The listing builds one solid part. Answer for the finished solid, in the listing's coordinates (mm). Coordinates: 2 decimals unless noted, no trailing zeros. Order: outer loops, then holes, each group sorted by start corner. A loop starts at its lowest first (then second) coordinate and runs counter-clockwise, first axis right, second up. Notation, with made-up numbers: (5.5, 81.25) -> (15.5, 81.25) arc R9 ccw to (15.5, 95.25) -> close; hole circle Ø3 at (61, 82.25). An arc over 180 degrees is marked (long way). Answer in a Markdown table with one row per item.
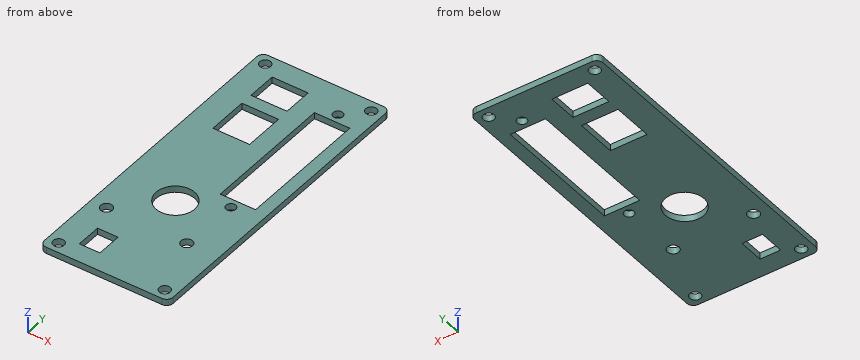
```python
from build123d import *

# Parameters (mm, degrees)
SKETCH_W      = 40
SKETCH_H      = 96.5
PAD_DEPTH     = 2
SKETCH001_R   = 1.7
SKETCH001_R_2 = 1.5
SKETCH001_R_3 = 6
SKETCH001_R_4 = 1.8
SKETCH001_W   = 11
SKETCH001_H   = 41
SKETCH001_W_2 = 11.2
SKETCH001_H_2 = 9.2
SKETCH001_W_3 = 11.4
SKETCH001_H_3 = 12.6
SKETCH001_W_4 = 6.4
SKETCH001_H_4 = 7.9
POCKET_DEPTH  = 5
FILLET_R      = 2
FILLET001_R   = 2
FILLET002_R   = 2
FILLET003_R   = 2


with BuildPart() as part:
    # Sketch → Pad (new body)
    with BuildSketch(Plane.XY):
        Rectangle(SKETCH_W, SKETCH_H)
    extrude(amount=PAD_DEPTH)

    # Sketch001 (on Face6 of Pad) → Pocket (cut)
    with BuildSketch(Plane.XY.offset(2)):
        with Locations((-16.5, 44.95)):
            Circle(SKETCH001_R)
        with Locations((16.5, 44.95)):
            Circle(SKETCH001_R)
        with Locations((-16.5, -44.95)):
            Circle(SKETCH001_R)
        with Locations((16.5, -44.95)):
            Circle(SKETCH001_R)
        with Locations((10.5, 38.85)):
            Circle(SKETCH001_R_2)
        with Locations((10.5, -7.75)):
            Circle(SKETCH001_R_2)
        with Locations((-2.5, -13.75)):
            Circle(SKETCH001_R_3)
        with Locations((-15, -26.25)):
            Circle(SKETCH001_R_4)
        with Locations((10, -26.25)):
            Circle(SKETCH001_R_4)
        with Locations((10.68, 15.55)):
            Rectangle(SKETCH001_W, SKETCH001_H)
        with Locations((-6.4, 37.05754)):
            Rectangle(SKETCH001_W_2, SKETCH001_H_2)
        with Locations((-6.3, 22.205288)):
            Rectangle(SKETCH001_W_3, SKETCH001_H_3)
        with Locations((-8.8, -38.3)):
            Rectangle(SKETCH001_W_4, SKETCH001_H_4)
    extrude(amount=-POCKET_DEPTH, mode=Mode.SUBTRACT)

    # Fillet
    fillet_edges = [part.edges().sort_by_distance(p)[0] for p in [
        (-20, 48.25, 1),
    ]]
    fillet(fillet_edges, radius=FILLET_R)

    # Fillet001
    fillet001_edges = [part.edges().sort_by_distance(p)[0] for p in [
        (20, 48.25, 1),
    ]]
    fillet(fillet001_edges, radius=FILLET001_R)

    # Fillet002
    fillet002_edges = [part.edges().sort_by_distance(p)[0] for p in [
        (-20, -48.25, 1),
    ]]
    fillet(fillet002_edges, radius=FILLET002_R)

    # Fillet003
    fillet003_edges = [part.edges().sort_by_distance(p)[0] for p in [
        (20, -48.25, 1),
    ]]
    fillet(fillet003_edges, radius=FILLET003_R)


solid = part.part
```
(1) A cutting plane is placed at C-C, the plane x = 2. Determine the outline of the cut face in (y, z), then the cut area to 3 significant figures.
Check values:
| item | result |
|---|---|
| outline | (-48.25, 0) -> (-17.72, 0) -> (-17.72, 2) -> (-48.25, 2) -> close; (-9.78, 0) -> (48.25, 0) -> (48.25, 2) -> (-9.78, 2) -> close |
| area | 177 mm² |
(2) A cutting plane is placed at A-A, the plane y = 44.95. Determine the outline of the cut face in (x, z).
Check values:
| item | result |
|---|---|
| outline | (-20, 0) -> (-18.2, 0) -> (-18.2, 2) -> (-20, 2) -> close; (-14.8, 0) -> (14.8, 0) -> (14.8, 2) -> (-14.8, 2) -> close; (18.2, 0) -> (20, 0) -> (20, 2) -> (18.2, 2) -> close |
(3) A cutting plane is placed at D-D, the plane z = 1.1. Count the separate pieces of the cut face and the enclosed holes in it, then the cut area to 3 significant figures.
Check values:
| item | result |
|---|---|
| separate pieces | 1 |
| enclosed holes | 13 |
| area | 2,920 mm² |
(4) Find the intervals of material crossed by line 1 along X through (y, z) = (22, 1.7); line 2 along Y through (x, z) = (-2.5, 0.7); line 3 along Y through (x, z) = (-9.5, 1.95), in increasing order. Write a range as from..to.
Check values:
| item | result |
|---|---|
| line 1 | -20..-12, -0.6..5.18, 16.18..20 |
| line 2 | -48.25..-19.75, -7.75..15.91, 28.51..32.46, 41.66..48.25 |
| line 3 | -48.25..-42.25, -34.35..15.91, 28.51..32.46, 41.66..48.25 |
(5) A flat-ended cylindrical pin translates along its axis: pin 1 (9.5 mm diameter, centred on x = -2.5, y = -13.75, fed in from +Z). Find the tip coordinate at first contact, or state that the pin passes through.
Check values:
| item | result |
|---|---|
| pin 1 | through |
(6) A cutting plane is placed at B-B, the plane y = -13.75. Determine the outline of the cut face in (x, z), then the cut area to 3 significant figures.
Check values:
| item | result |
|---|---|
| outline | (-20, 0) -> (-8.5, 0) -> (-8.5, 2) -> (-20, 2) -> close; (3.5, 0) -> (20, 0) -> (20, 2) -> (3.5, 2) -> close |
| area | 56.0 mm² |
